Work out the finished part from the listing and answer in its coordinate system (mm). Face numbers are marked on the shaded views. A direction names the side the tool comes from. Coordinates: 2 decimals unless noted, no trailing zeros. Order: outer loops, then holes, each group sorted by start corner. A loop starts at its lowest first (then second) coordinate and runs counter-clockwise, first axis right, second up. Notation, with made-up numbers: (69.25, 86.25) - (113.25, 86.25) arc R18 cw to (113.25, 101.25) - close; hole circle Ø5 at (28.25, 80.5). An arc over 180 degrees is marked (long way). Answer as a JSON object with one key per item and string values. Group by question number.
1) Section B-B (x = -9) is taken. Give the vertices of the cut face in (y, z).
2) Each of these flat-tipped pins is pushed along its axis until it touches: P1, Ø4, axis at y = -20.5, z = -7, coming from the -X side; P2, Ø0.5, axis at x = 4, z = -7, coming from the -Y side; P3, Ø2, axis at x = -7, y = -12.5, coming from the -Z side. Where does it stop, or does it pass through?
3) Section A-A (z = 0) is taken. Count the separate pieces of the cut face and the enclosed holes in it, plus the area to 3 significant figures.
4) A tool of negligible diameter and unlimited length cuts with its end or side. For the marked faces 1, 2, 3 and 4, from which of +Z, -Z, +X, -X, +Y, -Y can it reach the whole face along a straight path? Write none if from no direction.
5) The mould has two halves that part along Y. Classify the marked faces 5, 6, 7 and 8: released by +Y, released by -Y, zero draft, split by the parting line, or undercut.
6) Section C-C (x = 0) is taken. Give the vertices of the cut face in (y, z), plus the area to 3 significant figures.
7) Find the intervals of material crossed by line 1 along Y through (x, z) = (1, 9.25); line 2 along Y through (x, z) = (-0.5, -2.25); line 3 along X through (y, z) = (-9, 0), in increasing order.
8) Section D-D (y = -5.5) is taken. Give the vertices of the cut face in (x, z).
from build123d import *

# Parameters (mm, degrees)
F0_R          = 10.8
F0_R_2        = 5
F1_DEPTH      = 30
F2_DEPTH      = 15
F3_R          = 1.65
F4_DEPTH      = 10.801
F4_DEPTH_BACK = 10.801
F6_R          = 10.8
F6_R_2        = 8.25
F7_DEPTH      = 3.5
F8_R          = 1.25
F9_DEPTH      = 3


with BuildPart() as f1:
    # F0 (on Front) → F1 (new body)
    with BuildSketch(Plane.XZ):
        Circle(F0_R)
        Circle(F0_R_2, mode=Mode.SUBTRACT)
        Circle(F0_R_2)
    extrude(amount=F1_DEPTH)

    # F0 (on Front) → F2 (cut)
    with BuildSketch(Plane.XZ):
        Circle(F0_R_2)
    extrude(amount=F2_DEPTH, mode=Mode.SUBTRACT)

    # F3 (on Right) → F4 (cut, two sides)
    with BuildSketch(Plane.YZ) as f4_sk:
        with Locations((-6, 0)):
            Circle(F3_R)
    extrude(amount=-F4_DEPTH, mode=Mode.SUBTRACT)
    extrude(f4_sk.sketch, amount=F4_DEPTH_BACK, mode=Mode.SUBTRACT)

    # F6 (on offset) → F7 (cut)
    with BuildSketch(Plane.XZ.offset(28)):
        Circle(F6_R)
        Circle(F6_R_2, mode=Mode.SUBTRACT)
    extrude(amount=-F7_DEPTH, mode=Mode.SUBTRACT)

    # F8 (on face) → F9 (cut)
    with BuildSketch(Plane.XZ.offset(30)):
        with Locations((-4.125, 7.1447095812)):
            Circle(F8_R)
        with Locations((4.125, 7.1447095812)):
            Circle(F8_R)
        with Locations((-8.25, 0)):
            Circle(F8_R)
        with Locations((-4.125, -7.1447095812)):
            Circle(F8_R)
        with Locations((4.125, -7.1447095812)):
            Circle(F8_R)
        with Locations((8.25, 0)):
            Circle(F8_R)
    extrude(amount=-F9_DEPTH, mode=Mode.SUBTRACT)


solid = f1.part
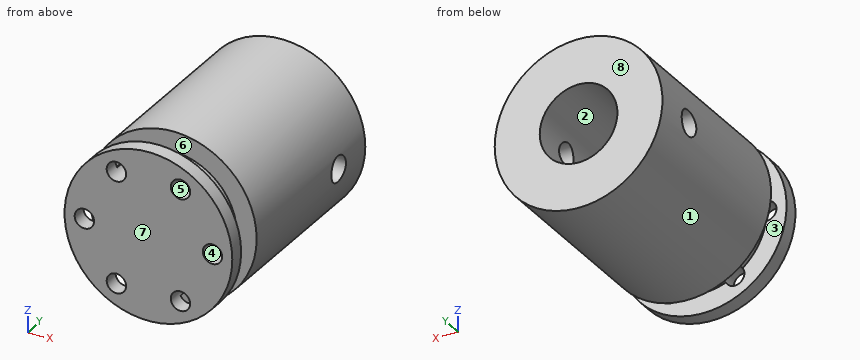
Report:
{
 "1": {"outline": "(-30, -5.97) - (-28, -5.97) - (-28, -1) - (-30, -1) - close; (-30, 1) - (-28, 1) - (-28, 5.97) - (-30, 5.97) - close; (-24.5, -5.97) - (0, -5.97) - (0, 5.97) - (-24.5, 5.97) - close; hole circle Ø3.3 at (-6, 0)"},
 "2": {"P1": "stops at x = -9.57", "P2": "stops at y = -27", "P3": "stops at z = -8.98"},
 "3": {"separate pieces": "5", "enclosed holes": "0", "area": "429 mm²"},
 "4": {"face 1": "+Y, -Y", "face 2": "+Y", "face 3": "none", "face 4": "-Y"},
 "5": {"face 5": "zero draft", "face 6": "undercut", "face 7": "released by -Y", "face 8": "released by +Y"},
 "6": {"outline": "(-30, -10.8) - (-28, -10.8) - (-28, -8.25) - (-24.5, -8.25) - (-24.5, -10.8) - (0, -10.8) - (0, -5) - (-15, -5) - (-15, 5) - (0, 5) - (0, 10.8) - (-24.5, 10.8) - (-24.5, 8.25) - (-28, 8.25) - (-28, 10.8) - (-30, 10.8) - close", "area": "480 mm²"},
 "7": {"line 1": "y = -30 to -28, -24.5 to 0", "line 2": "y = -30 to -15", "line 3": "x = -10.8 to -5, 5 to 10.8"},
 "8": {"outline": "(-10.68, -1.57) arc R10.8 ccw to (10.68, -1.57) - (4.75, -1.57) arc R5 cw to (-4.75, -1.57) - close; (-10.68, 1.57) - (-4.75, 1.57) arc R5 cw to (4.75, 1.57) - (10.68, 1.57) arc R10.8 ccw to start"}
}
